Verification items for the finished model (mm, model axes). A direction names the side the tool comes from. Coordinates: 2 decimals unless noted, no trailing zeros. Write each loop counter-clockwise with the first axis right and the second up, starting at its lowest first coordinate (ties: lowest second). Pieces come first, ordered by that corner, then holes. Notation, with made-up numbers: M 18.25,22 L 53.25,22 A30 ccw 53.25,46 Z; hole C 80.25,64 d8. An arc over 180 degrees is marked long. One line per item, written item: value.
Autodesk Inventor part; units mm, degrees
ref_plane "YZ Plane" through (0, 0, 0) normal (1, 0, 0) x (0, 1, 0)
ref_plane "XZ Plane" through (0, 0, 0) normal (0, 1, 0) x (-1, 0, 0)
ref_plane "XY Plane" through (0, 0, 0) normal (0, 0, 1) x (1, 0, 0)
sketch "Sketch1" plane through (0, 0, 0) normal (0, 1, 0) x (-1, 0, 0)
  line L0 (0, 0) -> (25.4, 0)
  line L1 (25.4, 0) -> (25.4, -25.4)
  line L2 (25.4, -25.4) -> (0, -25.4)
  line L3 (0, -25.4) -> (0, 0)
  line L4 (23.8125, -1.5875) -> (1.5875, -1.5875)
  line L5 (1.5875, -1.5875) -> (1.5875, -23.8125)
  line L6 (1.5875, -23.8125) -> (23.8125, -23.8125)
  line L7 (23.8125, -23.8125) -> (23.8125, -1.5875)
  dimension "d0" = 25.4
  dimension "d1" = 25.4
  dimension "d2" = 1.5875
extrude "Extrusion1" add sketch "Sketch1" along normal blind 473.075
chamfer "Chamfer1" distance 25.4 angle 45 1 edges at (0, 473.075, -12.7)
properties part number "SUP_001_CornerVertical" material "Aluminum 6061"
Item 1: Cross-section at B-B, the plane y = 356. Enter the section's corners in (x, z), and give its area (3 significant figures).
The answers:
outline: M -25.4,-25.4 L 0,-25.4 L 0,0 L -25.4,0 Z; hole M -23.81,-23.81 L -1.59,-23.81 L -1.59,-1.59 L -23.81,-1.59 Z
area: 151 mm²
Item 2: Cross-section at A-A, the plane z = -9.5. Enter the section's corners in (x, y) (1 decimal).
The answers:
outline: M -25.4,0 L -23.8,0 L -23.8,471.5 L -25.4,473.1 Z; M -1.6,0 L 0,0 L 0,447.7 L -1.6,449.3 Z
Item 3: Cross-section at C-C, the plane x = -17.75. Enter the section's corners in (y, z) (1 decimal).
The answers:
outline: M 0,-25.4 L 465.4,-25.4 L 465.4,-23.8 L 0,-23.8 Z; M 0,-1.6 L 465.4,-1.6 L 465.4,0 L 0,0 Z
Item 4: Scan lines: line 1 (Z direction, x = -23.5, y = 424.5); line 2 (Y direction, x = -10.5, z = -1.5) (3 decimals). Record each from-to range of solid material in increasing order.
The answers:
line 1: z = -25.4 to -23.81, -1.59 to 0
line 2: y = 0 to 458.175
Item 5: Access from +Z, -Z, +X, -X, +Y, -Y to the whole of each face (thin tool, end or side, straight path). Record for faces 1 (the face through (0, 221, -13)), 2 (the face through (-13, 232, -1.588)).
The answers:
face 1: +Z, -Z, +X, +Y, -Y
face 2: +Y, -Y
Item 6: Draft check along Z on faces 3 (the face through (-12.641, 460.316, -24.048)), 4 (the face through (-1.588, 221, -13)), 5 (the face through (-13, 233, 0)). Enter one of: released by +Z, released by -Z, zero draft, split by the parting line, or undercut.
The answers:
face 3: zero draft
face 4: undercut
face 5: released by +Z
